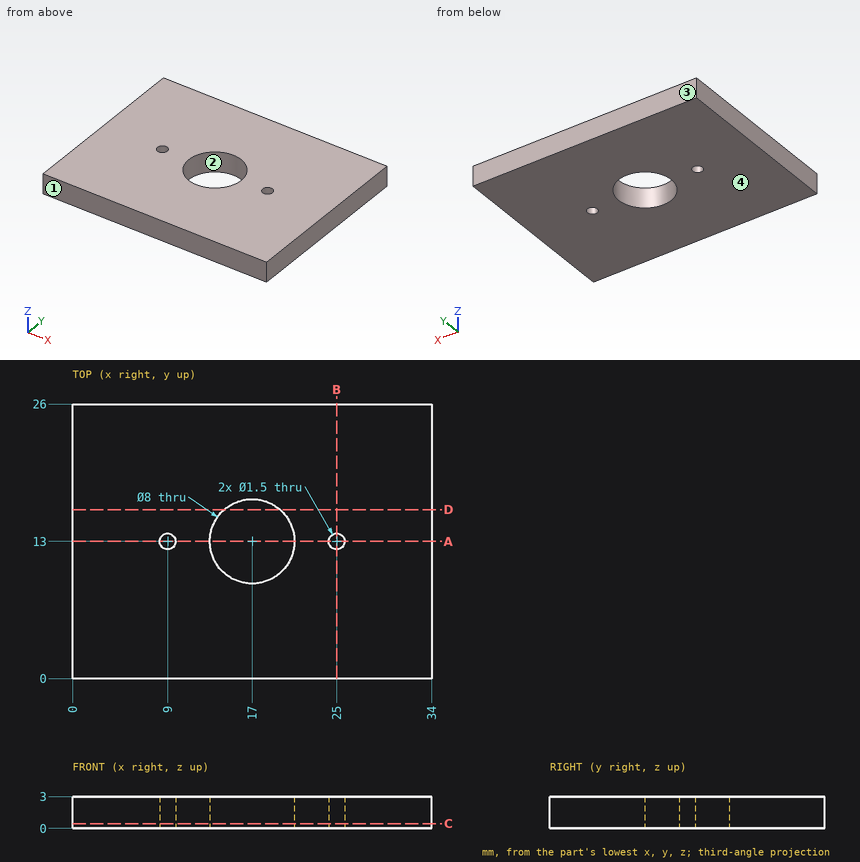
Design review of the part shown in the three views and the two pictorial views. Dimensions are in mm from the part's minimum x, y and z. Coordinates: 2 decimals unless noted, no trailing zeros. Loops run counter-clockwise (first coordinate to the right, second up) from the corner with the lowest first, then second, coordinate; pieces in that order, holes last. Notation, with made-up numbers: (-34, 25) -> (-22, 25) arc R18 ccw to (-22, 51) -> close; hole circle Ø1 at (21, -23). An arc over 180 degrees is marked (long way). Answer as CSV lines item,"result".
Item 1: Take a section at B-B, the plane x = 25. State the section outline as (y, z) points.
Results below:
outline,"(0, 0) -> (12.25, 0) -> (12.25, 3) -> (0, 3) -> close; (13.75, 0) -> (26, 0) -> (26, 3) -> (13.75, 3) -> close"
Item 2: Take a section at C-C, the plane z = 0.45. State the section outline as (x, y) points.
Results below:
outline,"(0, 0) -> (34, 0) -> (34, 26) -> (0, 26) -> close; hole circle Ø1.5 at (9, 13); hole circle Ø8 at (17, 13); hole circle Ø1.5 at (25, 13)"
Item 3: Take a section at A-A, the plane y = 13. State the section outline as (x, z) points, and give its area (3 significant figures).
Results below:
outline,"(0, 0) -> (8.25, 0) -> (8.25, 3) -> (0, 3) -> close; (9.75, 0) -> (13, 0) -> (13, 3) -> (9.75, 3) -> close; (21, 0) -> (24.25, 0) -> (24.25, 3) -> (21, 3) -> close; (25.75, 0) -> (34, 0) -> (34, 3) -> (25.75, 3) -> close"
area,"69.0 mm2"
Item 4: Draft analysis for pull direction Y (two halves, no side actions). For the marked faces 1, 2, 3 and 4, state which applies: +Y half, -Y half, draft (parallel to the pull), parting line (faces both ways), or undercut.
Results below:
face 1,"-Y half"
face 2,"undercut"
face 3,"+Y half"
face 4,"draft"
Item 5: For L1, parallel to X at y = 13, z = 1.6; L2, parallel to Y at x = 25, z = 1.25; L3, parallel to X at y = 12.5, z = 2.75, list the stretches that pass through material, from the lowest coordinate up.
Results below:
L1,"x = 0 to 8.25, 9.75 to 13, 21 to 24.25, 25.75 to 34"
L2,"y = 0 to 12.25, 13.75 to 26"
L3,"x = 0 to 8.44, 9.56 to 13.03, 20.97 to 24.44, 25.56 to 34"
Item 6: Take a section at D-D, the plane y = 16. State the section outline as (x, z) points, and give its area (3 significant figures).
Results below:
outline,"(0, 0) -> (14.35, 0) -> (14.35, 3) -> (0, 3) -> close; (19.65, 0) -> (34, 0) -> (34, 3) -> (19.65, 3) -> close"
area,"86.1 mm2"
Item 7: Insertion check: pin 1 (7 mm diameter, centred on x = 17, y = 13, fed in from -Z). The pin has a flat end and moves straight along its axis. Give the tip position at first contact, or say it passes through.
Results below:
pin 1,"passes through"
